Source: three-view drawing plus pictorial views. Frame: mm from the lowest corner of the part. A direction names the side the tool comes from. Round coordinates to 2 decimals unless told otherwise and drop trailing zeros. Write each loop counter-clockwise with the first axis right and the second up, starting at its lowest first coordinate (ties: lowest second). Pieces come first, ordered by that corner, then holes.
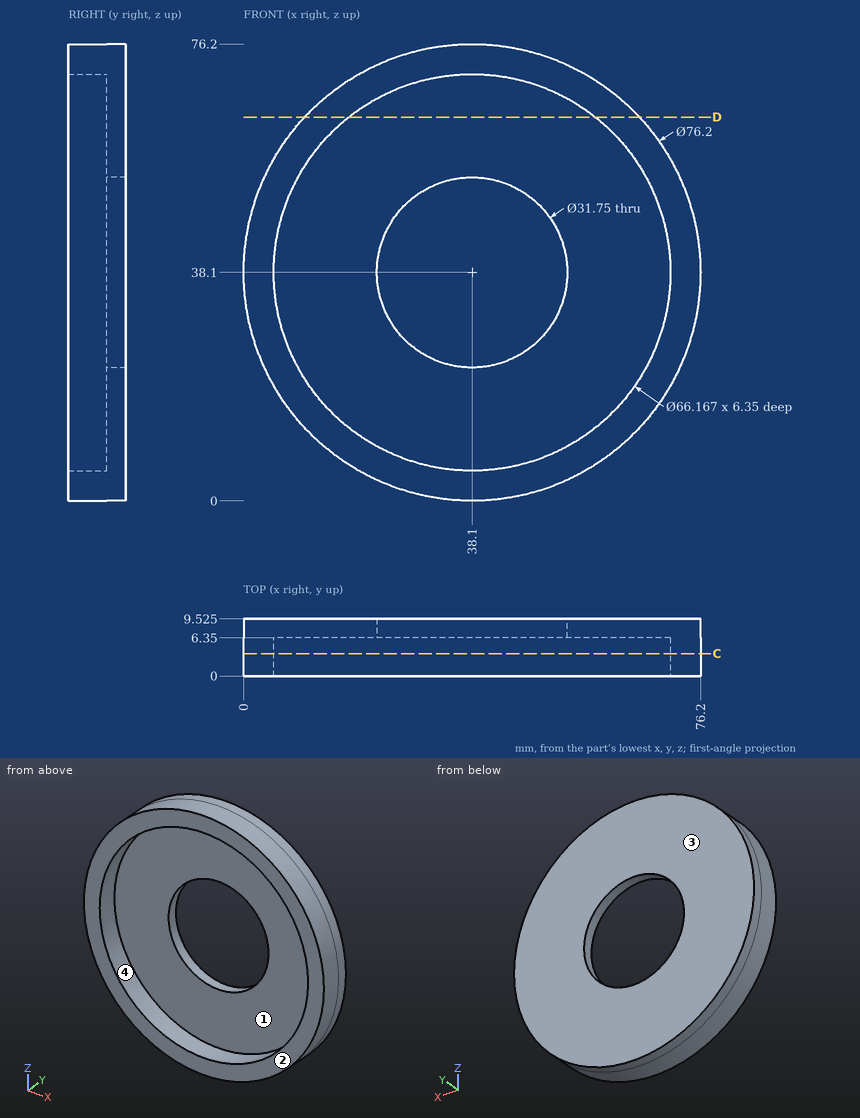
1) Section D-D on z = 64. Output: boundary loops of the cut face in (x, y) (3 decimals).
2) Section C-C on y = 3.75. Output: boundary loops of the cut face in (x, z).
3) First-contact query: P1, Ø2, axis at x = 49, y = 7, coming from the +Z side; P2, Ø4, axis at x = 30.5, y = 1.5, coming from the +Z side; P3, Ø2, axis at x = 51, z = 41, coming from the +Y side; P4, Ø3, axis at x = 32, y = 2.5, coming from the +Z side. Flat tips, straight axial feed; report the tip coordinate or a pass-through.
4) Draft query along X for the marked faces 3 and 4. Return one class per face: pulls with the +X half, pulls with the -X half, needs draft (parallel to the pull), parting line crosses it, or undercut.
5) Line query: probe 1 along Z at (x, y) = (38.1, 4.5); probe 2 along Z at (x, y) = (38.1, 8.8) (3 decimals). Output: solid intervals per line, ascending.
6) Reachability of the marked faces 1 and 2 from +Z, -Z, +X, -X, +Y, -Y: full face, straight path, thin tool, end or side. Return the list, or none.
Filled in:
1. outline: (10.157, 0) - (17.516, 0) - (17.516, 6.35) - (58.684, 6.35) - (58.684, 0) - (66.043, 0) - (66.043, 9.525) - (10.157, 9.525) - close
2. outline: circle Ø76.2 at (38.1, 38.1); hole circle Ø66.17 at (38.1, 38.1)
3. P1: stops at z = 74.89
3. P2: stops at z = 75.79
3. P3: passes through
3. P4: stops at z = 75.92
4. face 3: needs draft
4. face 4: undercut
5. probe 1: z = 0 to 5.02, 71.18 to 76.2
5. probe 2: z = 0 to 22.225, 53.975 to 76.2
6. face 1: -Y
6. face 2: +Z, -Z, +X, -X, -Y
